Drawing for the job (mm, zero at the part's lowest x, y, z). A direction names the side the tool comes from. Round coordinates to 2 decimals unless told otherwise and drop trailing zeros. Loops run counter-clockwise (first coordinate to the right, second up) from the corner with the lowest first, then second, coordinate; pieces in that order, holes last. Notation, with made-up numbers: M 24.25,67 L 54.25,67 A8 cw 54.25,78 Z; hole C 80,-23 d8. An arc over 180 degrees is marked long. Use a Markdown table: item, result. Add a question column.
Q1. Cut at D-D (z = 4). Give the cut face in (x, y).
Q2. Pin check, flat tips, straight feed: pin 1 (0.9 mm diameter, centred on y = 71.5, z = 8.5, fed in from -X); pin 2 (3 mm diameter, centred on x = 19.5, y = 43, fed in from +Z); pin 3 (2.5 mm diameter, centred on y = 47.5, z = 9, fed in from +X). Stop position of each tip, or through.
Q3. Tool access for the marked faces 1 and 2: list every direction of +Z, -Z, +X, -X, +Y, -Y with a clear straight run to the whole face (end or side of a thin tool).
Q4. Mould opens along Y. For the marked faces 3, 4 and 5 say: +Y half, -Y half, draft (parallel to the pull), parting line (faces both ways), or undercut.
Q5. Cut at B-B (y = 44.5). Give the cut face in (x, z).
Q6. Cut at A-A (z = 8.75). Give the cut face in (x, y), plus the area to 3 significant figures.
Q7. Probe line 1 (Y direction, x = 9.5, z = 7); line 2 (Y direction, x = 5, z = 5); line 3 (Z direction, x = 33, y = 75.5). List the from-to ranges inside material, lowest first. Write a range as from..to.
Q8. Cut at C-C (x = 33). Give the cut face in (y, z).
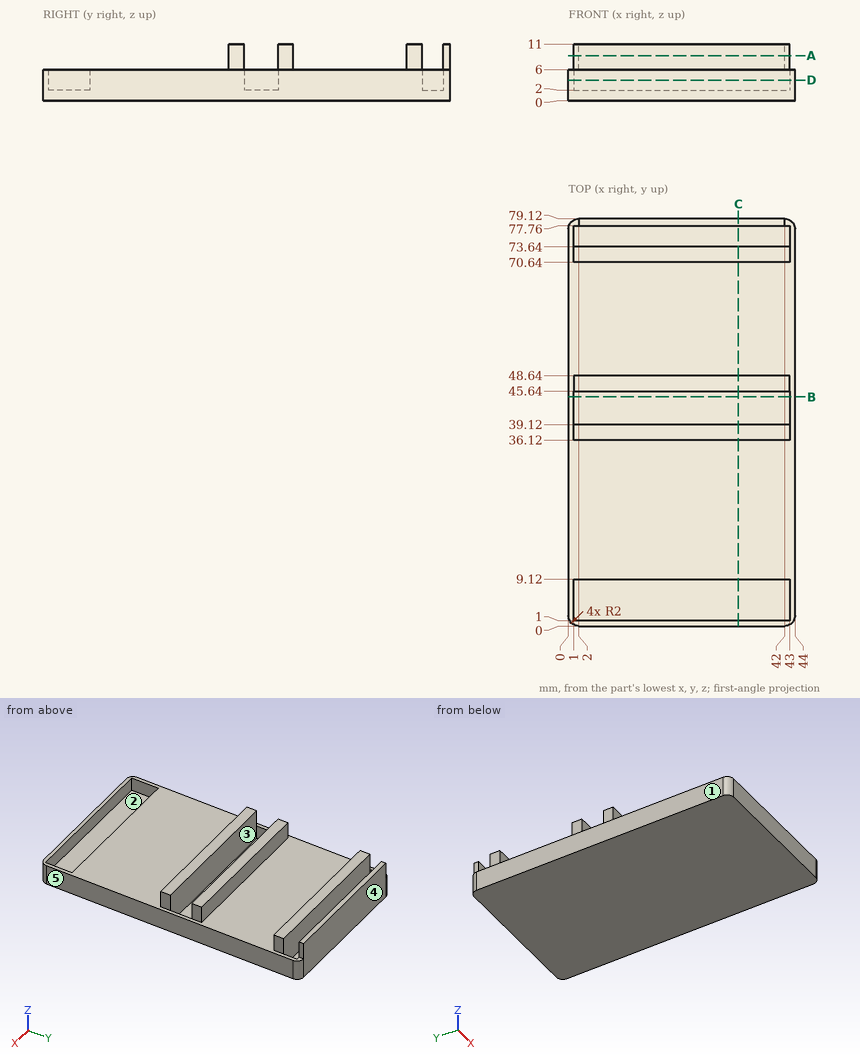
Checked values:
| question | item | result |
|---|---|---|
| 1 | outline | M 0,2 A2 ccw 2,0 L 42,0 A2 ccw 44,2 L 44,77.12 A2 ccw 42,79.12 L 2,79.12 A2 ccw 0,77.12 Z; hole M 1,1 L 43,1 L 43,9.12 L 1,9.12 Z; hole M 1,39.12 L 43,39.12 L 43,45.64 L 1,45.64 Z; hole M 1,73.64 L 43,73.64 L 43,77.76 L 1,77.76 Z |
| 2 | pin 1 | stops at x = 1 |
| 2 | pin 2 | stops at z = 2 |
| 2 | pin 3 | stops at x = 43 |
| 3 | face 1 | +Z, -Z, -X, +Y, -Y |
| 3 | face 2 | +Z |
| 4 | face 3 | undercut |
| 4 | face 4 | +Y half |
| 4 | face 5 | draft |
| 5 | outline | M 0,0 L 44,0 L 44,6 L 43,6 L 43,2 L 1,2 L 1,6 L 0,6 Z |
| 6 | outline | M 1,36.12 L 43,36.12 L 43,39.12 L 1,39.12 Z; M 1,45.64 L 43,45.64 L 43,48.64 L 1,48.64 Z; M 1,70.64 L 43,70.64 L 43,73.64 L 1,73.64 Z; M 2,77.76 L 42,77.76 L 42,79.12 L 2,79.12 Z |
| 6 | area | 432 mm^2 |
| 7 | line 1 | y = 36.12..39.12, 45.64..48.64, 70.64..73.64, 77.76..79.12 |
| 7 | line 2 | y = 0..1, 9.12..39.12, 45.64..73.64, 77.76..79.12 |
| 7 | line 3 | z = 0..2 |
| 8 | outline | M 0,0 L 79.12,0 L 79.12,11 L 77.76,11 L 77.76,2 L 73.64,2 L 73.64,11 L 70.64,11 L 70.64,6 L 48.64,6 L 48.64,11 L 45.64,11 L 45.64,2 L 39.12,2 L 39.12,11 L 36.12,11 L 36.12,6 L 9.12,6 L 9.12,2 L 1,2 L 1,6 L 0,6 Z |
